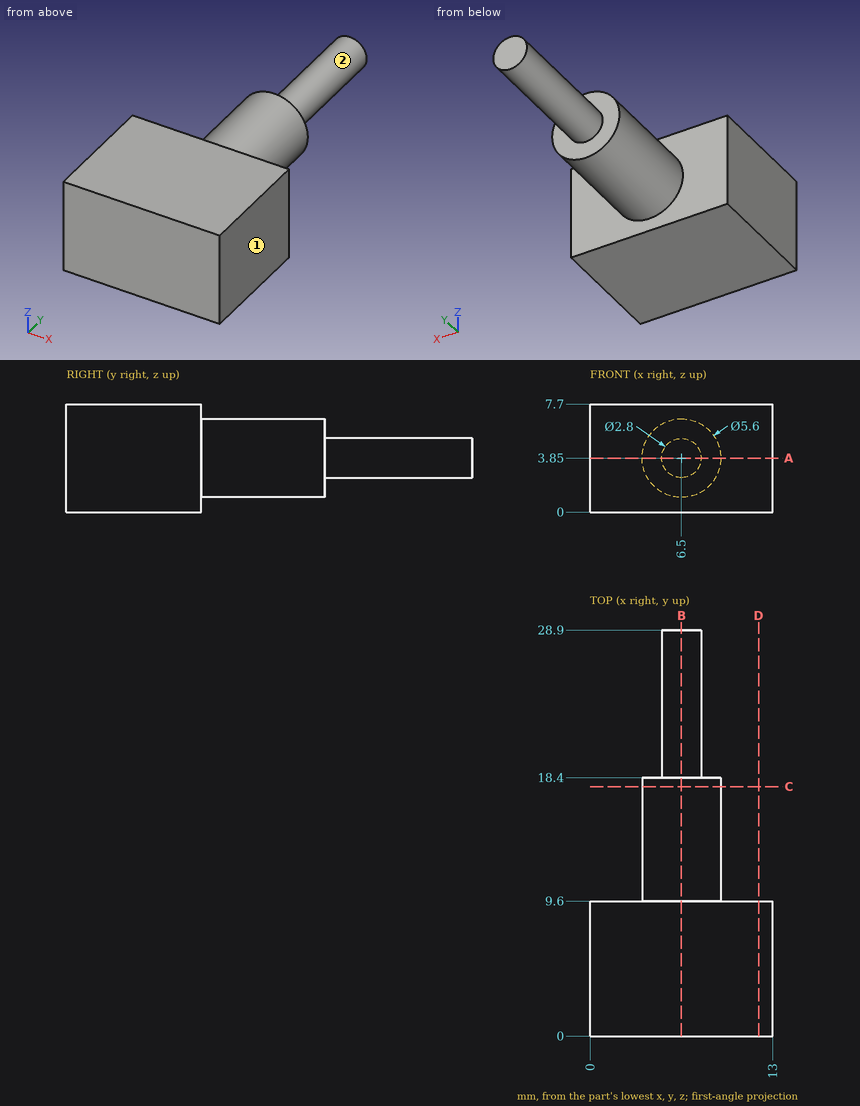
The drawing under review shows one solid part. Ordinate dimensions are in mm from its lowest x, y, z. A direction names the side the tool comes from. Round coordinates to 2 decimals unless told otherwise and drop trailing zeros. Write each loop counter-clockwise with the first axis right and the second up, starting at its lowest first coordinate (ties: lowest second). Pieces come first, ordered by that corner, then holes. Notation, with made-up numbers: (-33.75, -6.75) - (-24.75, -6.75) arc R17 cw to (-24.75, 20.25) - close; hole circle Ø5 at (-27, -36). An arc over 180 degrees is marked (long way). Use a Markdown table: item, result. Add a question column.
1. Wall thickness on probe 1 along Y at (x, z) = (3.5, 3); probe 2 along Y at (x, z) = (8.5, 5.25); probe 3 along Z at (x, y) = (6.5, 20.75): over which ranges is each line inside the solid? List them lowest first.
2. For the marked faces 1 and 2, list the 3-axis set-ups (+Z, -Z, +X, -X, +Y, -Y) from which the entire face can be reached by the end or side of a thin tool; tool diameter is ignored.
3. We need section B-B (x = 6.5). State the section outline as (y, z) points.
4. We need section D-D (x = 12). State the section outline as (y, z) points, then the cut area to 3 significant figures.
5. Clearance check with a flat-ended pin moving along its axis: pin 1 (2 mm diameter, centred on y = 5, z = 1.5, fed in from -X). State where the tip first meets the part, or that it passes through.
6. We need section C-C (y = 17.75). State the section outline as (x, z) points, then the cut area to 3 significant figures.
7. We need section A-A (z = 3.85). State the section outline as (x, y) points.
Output:
| question | item | result |
|---|---|---|
| 1 | probe 1 | y = 0 to 9.6 |
| 1 | probe 2 | y = 0 to 18.4 |
| 1 | probe 3 | z = 2.45 to 5.25 |
| 2 | face 1 | +Z, -Z, +X, +Y, -Y |
| 2 | face 2 | +Y |
| 3 | outline | (0, 0) - (9.6, 0) - (9.6, 1.05) - (18.4, 1.05) - (18.4, 2.45) - (28.9, 2.45) - (28.9, 5.25) - (18.4, 5.25) - (18.4, 6.65) - (9.6, 6.65) - (9.6, 7.7) - (0, 7.7) - close |
| 4 | outline | (0, 0) - (9.6, 0) - (9.6, 7.7) - (0, 7.7) - close |
| 4 | area | 73.9 mm2 |
| 5 | pin 1 | stops at x = 0 |
| 6 | outline | circle Ø5.6 at (6.5, 3.85) |
| 6 | area | 24.6 mm2 |
| 7 | outline | (0, 0) - (13, 0) - (13, 9.6) - (9.3, 9.6) - (9.3, 18.4) - (7.9, 18.4) - (7.9, 28.9) - (5.1, 28.9) - (5.1, 18.4) - (3.7, 18.4) - (3.7, 9.6) - (0, 9.6) - close |
